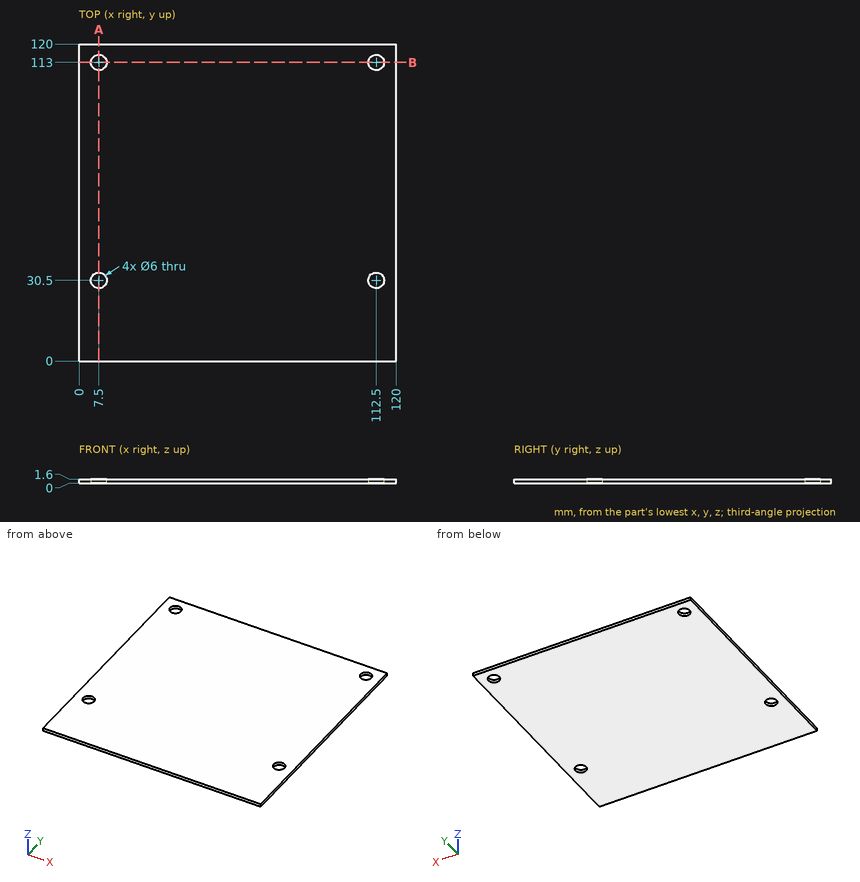
Source: three-view drawing plus pictorial views. Frame: mm from the lowest corner of the part. Round coordinates to 2 decimals unless told otherwise and drop trailing zeros. Loops run counter-clockwise (first coordinate to the right, second up) from the corner with the lowest first, then second, coordinate; pieces in that order, holes last.
Q1. Material intervals for L1, parallel to Y at x = 7.5, z = 1; L2, parallel to X at y = 113, z = 1.15; L3, parallel to X at y = 111.5, z = 0.8, sorted ascending.
Q2. Section B-B on y = 113. Return loops of the section in (x, z).
Q3. Pin query (flat end, axial travel): P1, Ø5, axis at x = 14, y = 90.5, coming from the -Z side. Return the tip coordinate at first contact, or that it passes through.
Q4. Section A-A on x = 7.5. Return loops of the section in (y, z), plus the area to 3 significant figures.
Evaluation:
1. L1: y = 0 to 27.5, 33.5 to 110, 116 to 120
1. L2: x = 0 to 4.5, 10.5 to 109.5, 115.5 to 120
1. L3: x = 0 to 4.9, 10.1 to 109.9, 115.1 to 120
2. outline: (0, 0) - (4.5, 0) - (4.5, 1.6) - (0, 1.6) - close; (10.5, 0) - (109.5, 0) - (109.5, 1.6) - (10.5, 1.6) - close; (115.5, 0) - (120, 0) - (120, 1.6) - (115.5, 1.6) - close
3. P1: stops at z = 0
4. outline: (0, 0) - (27.5, 0) - (27.5, 1.6) - (0, 1.6) - close; (33.5, 0) - (110, 0) - (110, 1.6) - (33.5, 1.6) - close; (116, 0) - (120, 0) - (120, 1.6) - (116, 1.6) - close
4. area: 173 mm2
